Verification items for the finished model (mm, model axes). A direction names the side the tool comes from. Coordinates: 2 decimals unless noted, no trailing zeros. Order: outer loops, then holes, each group sorted by start corner. A loop starts at its lowest first (then second) coordinate and runs counter-clockwise, first axis right, second up. Notation, with made-up numbers: M 77,-10.75 L 93,-10.75 A4 cw 93,-3.75 Z; hole C 44,-8 d11. An arc over 180 degrees is marked long. Return JSON: item names as keys, results as strings. Group by question number.
Q1. Go/stop test with flat-tipped pins: pin 1 Ø8 at (y, z) = (41, -2) entering from -X; pin 2 Ø1.5 at (x, z) = (-32, 0) entering from -Y; pin 3 Ø2 at (y, z) = (40, -5.5) entering from -X; pin 4 Ø2 at (x, z) = (-22.5, -5.5) entering from -Y. Record where each tip stops, or that it passes through.
Q2. Section check D-D, the plane x = -25. Enter the section's corners in (y, z), then the cut area to 3 significant figures.
Q3. Section check C-C, the plane y = 43.25. Enter the section's corners in (x, z), then the cut area to 3 significant figures.
Q4. Thickness scan on probe 1 along Z at (x, y) = (-32.75, 49.25); probe 2 along Y at (x, z) = (-21.5, -5.75); probe 3 along Y at (x, z) = (-21, 0.5). Record the ranges inside material, lowest first.
Q5. Mould release check, pull along Y, two halves, no side actions. Record for faces 3 (the face through (-35.603, 56, -4)), 4 (the face through (-25.383, 35.525, 1.479)), 5 (the face through (-20.834, 47.024, 1.479)), 6 (the face through (-20.834, 47.024, -9.479)): pulls with the +Y half, pulls with the -Y half, needs draft (parallel to the pull), parting line crosses it, or undercut.
Q6. Section check A-A, the plane x = -21.25. Enter the section's corners in (y, z).
Q7. Access from +Z, -Z, +X, -X, +Y, -Y to the whole of each face (thin tool, end or side, straight path). Record for faces 1 (the face through (-26, 55.523, -4)), 2 (the face through (-25.383, 35.525, -9.479)).
Q8. Section check B-B, the plane z = 2. Enter the section's corners in (x, y), then the cut area to 3 significant figures.
from build123d import *

# Parameters (mm, degrees)
SKETCH_1_R      = 5
EXTRUDE_1_DEPTH = 3
SKETCH_2_W      = 20
SKETCH_2_H      = 14
EXTRUDE_2_DEPTH = 3


with BuildPart() as part:
    # 草图1 → 凸台-拉伸1 (new body)
    with BuildSketch(Plane.XY):
        with BuildLine():
            Line((-35.60315534, 55.522572816), (-15.60315534, 55.522572816))
            Line((-15.60315534, 55.522572816), (-15.60315534, 45.522572816))
            ThreePointArc((-15.60315534, 45.522572816), (-25.60315534, 35.522572816), (-35.60315534, 45.522572816))
            Line((-35.60315534, 45.522572816), (-35.60315534, 55.522572816))
        make_face()
        with Locations((-25.60315534, 45.522572816)):
            Circle(SKETCH_1_R, mode=Mode.SUBTRACT)
    extrude_1 = extrude(amount=EXTRUDE_1_DEPTH)

    # 草图2 → 凸台-拉伸2 (add)
    with BuildSketch(Plane(origin=(0, 55.522572816, 0), x_dir=(1, 0, 0), z_dir=(0, 1, 0))):
        with Locations((-25.60315534, 4)):
            Rectangle(SKETCH_2_W, SKETCH_2_H)
    extrude(amount=EXTRUDE_2_DEPTH)

    # 镜向1: 凸台-拉伸1 across plane
    add(extrude_1.mirror(Plane(origin=(0, 0, -4), x_dir=(1, 0, 0), z_dir=(0, 0, -1))))


solid = part.part
Numbers:
{
 "1": {"pin 1": "stops at x = -35.55", "pin 2": "stops at y = 37.27", "pin 3": "passes through", "pin 4": "stops at y = 55.52"},
 "2": {"outline": "M 35.54,-11 L 40.56,-11 L 40.56,-8 L 35.54,-8 Z; M 35.54,0 L 40.56,0 L 40.56,3 L 35.54,3 Z; M 50.49,-11 L 58.52,-11 L 58.52,3 L 50.49,3 L 50.49,0 L 55.52,0 L 55.52,-8 L 50.49,-8 Z", "area": "102 mm2"},
 "3": {"outline": "M -35.34,-11 L -30.06,-11 L -30.06,-8 L -35.34,-8 Z; M -35.34,0 L -30.06,0 L -30.06,3 L -35.34,3 Z; M -21.15,-11 L -15.86,-11 L -15.86,-8 L -21.15,-8 Z; M -21.15,0 L -15.86,0 L -15.86,3 L -21.15,3 Z", "area": "63.4 mm2"},
 "4": {"probe 1": "z = -11 to -8, 0 to 3", "probe 2": "y = 55.52 to 58.52", "probe 3": "y = 36.65 to 43.57, 47.47 to 58.52"},
 "5": {"face 3": "needs draft", "face 4": "pulls with the -Y half", "face 5": "undercut", "face 6": "undercut"},
 "6": {"outline": "M 36.52,-11 L 43.06,-11 L 43.06,-8 L 36.52,-8 Z; M 36.52,0 L 43.06,0 L 43.06,3 L 36.52,3 Z; M 47.98,-11 L 58.52,-11 L 58.52,3 L 47.98,3 L 47.98,0 L 55.52,0 L 55.52,-8 L 47.98,-8 Z"},
 "7": {"face 1": "+X, -X, -Y", "face 2": "+Z, -Z, -Y"},
 "8": {"outline": "M -35.6,45.52 A10 ccw -15.6,45.52 L -15.6,58.52 L -35.6,58.52 Z; hole C -25.6,45.52 d10", "area": "339 mm2"}
}
